```python
from build123d import *

# Parameters (mm, degrees)
SKETCH1_R           = 17.25
BOSS_EXTRUDE1_DEPTH = 1.9
SKETCH2_R           = 14.75
BOSS_EXTRUDE2_DEPTH = 11.2
BOSS_EXTRUDE3_START = 1.9
SKETCH3_R           = 17.25
BOSS_EXTRUDE3_DEPTH = 1.9
SKETCH4_R           = 5
CUT_EXTRUDE1_DEPTH  = 29.637824638
SKETCH5_R           = 1.5
CUT_EXTRUDE2_DEPTH  = 29.637824638


with BuildPart() as part:
    # Sketch1 → Boss-Extrude1 (new body)
    with BuildSketch(Plane.XY):
        with Locations(Location((0, 0, 0), (0, 0, 180))):
            Circle(SKETCH1_R)
    extrude(amount=BOSS_EXTRUDE1_DEPTH)

    # Sketch2 → Boss-Extrude2 (add)
    with BuildSketch(Plane(origin=(0, 0, 0), x_dir=(-1, 0, 0), z_dir=(0, 0, -1))):
        Circle(SKETCH2_R)
    extrude(amount=BOSS_EXTRUDE2_DEPTH)

    # Sketch3 → Boss-Extrude3 (add)
    with BuildSketch(Plane(origin=(0, 0, -11.2), x_dir=(-1, 0, 0), z_dir=(0, 0, -1)).offset(BOSS_EXTRUDE3_START)):
        Circle(SKETCH3_R)
    extrude(amount=-BOSS_EXTRUDE3_DEPTH)

    # Sketch4 → Cut-Extrude1 (cut, through all)
    with BuildSketch(Plane(origin=(0, 0, -13.1), x_dir=(-1, 0, 0), z_dir=(0, 0, -1))):
        Circle(SKETCH4_R)
    extrude(amount=-CUT_EXTRUDE1_DEPTH, mode=Mode.SUBTRACT)

    # Sketch5 → Cut-Extrude2 (cut, through all)
    with BuildSketch(Plane(origin=(0, 0, -13.1), x_dir=(-1, 0, 0), z_dir=(0, 0, -1))):
        with Locations((0, 8.125)):
            Circle(SKETCH5_R)
        with Locations((8.125, 0)):
            Circle(SKETCH5_R)
        with Locations((0, -8.125)):
            Circle(SKETCH5_R)
        with Locations((-8.125, 0)):
            Circle(SKETCH5_R)
    extrude(amount=-CUT_EXTRUDE2_DEPTH, mode=Mode.SUBTRACT)


solid = part.part
```
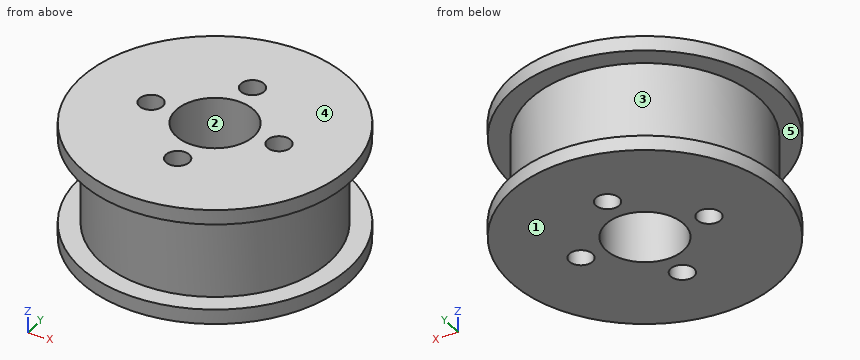
CAD build for the part. Positions are in the model's coordinates, mm. Face numbers are marked on the shaded views. A direction names the side the tool comes from. Round coordinates to 2 decimals unless told otherwise and drop trailing zeros. Write each loop counter-clockwise with the first axis right and the second up, starting at its lowest first coordinate (ties: lowest second). Pieces come first, ordered by that corner, then holes.
Item 1: Drill centre lines: L1, parallel to Y at x = 0, z = -1.5 (3 decimals); L2, parallel to Z at x = -9, y = 14; L3, parallel to Y at x = 0, z = 0.75 (3 decimals). Where is each one in solid material? Low to high.
Filled in:
L1: y = -14.75 to -9.625, -6.625 to -5, 5 to 6.625, 9.625 to 14.75
L2: z = -13.1 to -11.2, 0 to 1.9
L3: y = -17.25 to -9.625, -6.625 to -5, 5 to 6.625, 9.625 to 17.25
Item 2: Tool access for the marked faces 4 and 5: list every direction of +Z, -Z, +X, -X, +Y, -Y with a clear straight run to the whole face (end or side of a thin tool).
Filled in:
face 4: +Z, +X, -X, +Y, -Y
face 5: none
Item 3: Mould opens along Z. For the marked faces 1, 2 and 3 say: released by +Z, released by -Z, zero draft, split by the parting line, or undercut.
Filled in:
face 1: released by -Z
face 2: zero draft
face 3: undercut
Item 4: Drop flat-ended pins along their axis: pin 1 Ø2 at (y, z) = (-3.5, 0) entering from -X; pin 2 Ø2 at (x, y) = (-2, 2) entering from +Z; pin 3 Ø6 at (y, z) = (7, -3.5) entering from -X; pin 4 Ø2 at (x, z) = (10, -8) entering from -Y. Give the stop position or say it passes through.
Filled in:
pin 1: stops at x = -17.07
pin 2: passes through
pin 3: stops at x = -14.2
pin 4: stops at y = -11.69
Item 5: Band-saw the part on B-B on x = 15.5. Write the cut outline in (y, z), then the cut area to 3 significant figures.
Filled in:
outline: (-7.57, -13.1) - (7.57, -13.1) - (7.57, -11.2) - (-7.57, -11.2) - close; (-7.57, 0) - (7.57, 0) - (7.57, 1.9) - (-7.57, 1.9) - close
area: 57.5 mm2
Item 6: Band-saw the part on D-D on y = 13. Write the cut outline in (x, z).
Filled in:
outline: (-11.34, -13.1) - (11.34, -13.1) - (11.34, -11.2) - (6.97, -11.2) - (6.97, 0) - (11.34, 0) - (11.34, 1.9) - (-11.34, 1.9) - (-11.34, 0) - (-6.97, 0) - (-6.97, -11.2) - (-11.34, -11.2) - close
Item 7: Band-saw the part on A-A on y = 0. Write the cut outline in (x, z) (3 decimals).
Filled in:
outline: (-17.25, -13.1) - (-9.625, -13.1) - (-9.625, 1.9) - (-17.25, 1.9) - (-17.25, 0) - (-14.75, 0) - (-14.75, -11.2) - (-17.25, -11.2) - close; (-6.625, -13.1) - (-5, -13.1) - (-5, 1.9) - (-6.625, 1.9) - close; (5, -13.1) - (6.625, -13.1) - (6.625, 1.9) - (5, 1.9) - close; (9.625, -13.1) - (17.25, -13.1) - (17.25, -11.2) - (14.75, -11.2) - (14.75, 0) - (17.25, 0) - (17.25, 1.9) - (9.625, 1.9) - close
